```python
from build123d import *

# Parameters (mm, degrees)
PLUNGER_STEM_START     = 17.500063
SKETCH1_R              = 1.5
PLUNGER_STEM_DEPTH     = 26.499937
CAPTIVE_SHOULDER_START = 35.6
SKETCH2_R              = 2.4
CAPTIVE_SHOULDER_DEPTH = 1.2


with BuildPart() as part:
    # Sketch1 → Plunger_stem (new body)
    with BuildSketch(Plane.XY.offset(PLUNGER_STEM_START)):
        with Locations(Location((-32.018684277, -34.643402341, 0), (0, 0, 180))):
            Circle(SKETCH1_R)
    extrude(amount=PLUNGER_STEM_DEPTH)

    # Sketch2 → Captive_shoulder (add)
    with BuildSketch(Plane.XY.offset(CAPTIVE_SHOULDER_START)):
        with Locations((-32.018684277, -34.643402341)):
            Circle(SKETCH2_R)
    extrude(amount=CAPTIVE_SHOULDER_DEPTH)


solid = part.part
```
Geometry: final body of the model. Coordinates: model frame, mm. A direction names the side the tool comes from. Round coordinates to 2 decimals unless told otherwise and drop trailing zeros. Write each loop counter-clockwise with the first axis right and the second up, starting at its lowest first coordinate (ties: lowest second). Pieces come first, ordered by that corner, then holes. Notation, with made-up numbers: M -21.75,-19 L 7.25,-19 A33 cw 7.25,15 Z; hole C -6,54 d4. An arc over 180 degrees is marked long. Answer in a Markdown table with one row per item. Add a question column.
(1) Cut plane B-B, the plane x = -32.7. Return the cut outline in (y, z), then the cut area to 3 significant figures.
(2) Cut plane D-D, the plane x = -34.05. Return the cut outline in (y, z).
(3) Reachability of faces 1 (the face through (-30.913, -35.657, 40.35)), 2 (the face through (-32, -35, 44)), 3 (the face through (-30.913, -35.657, 26.423)) from +Z, -Z, +X, -X, +Y, -Y: full face, straight path, thin tool, end or side. Return the list, or none.
(4) Cut plane C-C, the plane z = 35.25. Return the cut outline in (x, y).
(5) Cut plane A-A, the plane y = -34.95. Return the cut outline in (x, z), then the cut area to 3 significant figures.
(6) Ray query, L1, parallel to Y at x = -31.9, z = 22.75; L2, parallel to Z at x = -33.8, y = -35.3; L3, parallel to Y at x = -31.4, z = 28.5. Return the intervals inside material, ascending.
Established:
| question | item | result |
|---|---|---|
| 1 | outline | M -36.94,35.6 L -35.98,35.6 L -35.98,17.5 L -33.31,17.5 L -33.31,35.6 L -32.34,35.6 L -32.34,36.8 L -33.31,36.8 L -33.31,44 L -35.98,44 L -35.98,36.8 L -36.94,36.8 Z |
| 1 | area | 73.1 mm² |
| 2 | outline | M -35.92,35.6 L -33.37,35.6 L -33.37,36.8 L -35.92,36.8 Z |
| 3 | face 1 | +Z |
| 3 | face 2 | +Z, +X, -X, +Y, -Y |
| 3 | face 3 | -Z |
| 4 | outline | C -32.02,-34.64 d3 |
| 5 | outline | M -34.4,35.6 L -33.49,35.6 L -33.49,17.5 L -30.55,17.5 L -30.55,35.6 L -29.64,35.6 L -29.64,36.8 L -30.55,36.8 L -30.55,44 L -33.49,44 L -33.49,36.8 L -34.4,36.8 Z |
| 5 | area | 80.0 mm² |
| 6 | L1 | -36.14 to -33.15 |
| 6 | L2 | 35.6 to 36.8 |
| 6 | L3 | -36.01 to -33.28 |
